```python
from build123d import *

# Parameters (mm, degrees)
SKETCH1_W             = 114.3
SKETCH1_H             = 25.4
SKETCH1_R             = 6.5
BOSS_EXTRUDE1_DEPTH   = 5.8
F_4_CLEARANCE_HOLE1_D = 2.9464
FILLET1_R             = 3.175


with BuildPart() as part:
    # Sketch1 → Boss-Extrude1 (new body)
    with BuildSketch(Plane(origin=(0, 0, 0), x_dir=(1, 0, 0), z_dir=(0, 1, 0))):
        with Locations((-57.15, 12.7)):
            Rectangle(SKETCH1_W, SKETCH1_H)
        with Locations(Location((-95.25, 12.7, 0), (0, 0, 270))):
            Circle(SKETCH1_R, mode=Mode.SUBTRACT)
        with Locations(Location((-57.15, 12.7, 0), (0, 0, 270))):
            Circle(SKETCH1_R, mode=Mode.SUBTRACT)
        with Locations(Location((-19.05, 12.7, 0), (0, 0, 270))):
            Circle(SKETCH1_R, mode=Mode.SUBTRACT)
    extrude(amount=BOSS_EXTRUDE1_DEPTH)

    # #4 Clearance Hole1 (through all)
    with Locations(Plane(origin=(0, 5.8, 0), x_dir=(-1, 0, 0), z_dir=(0, 1, 0))):
        with Locations((107.95, -22.225), (107.95, -3.175), (76.2, -22.225), (76.2, -3.175), (6.35, -22.225), (38.1, -22.225), (38.1, -3.175), (6.35, -3.175)):
            Hole(F_4_CLEARANCE_HOLE1_D / 2)

    # Fillet1
    fillet1_edges = [part.edges().sort_by_distance(p)[0] for p in [
        (0, 2.9, 0),
        (-114.3, 2.9, 0),
        (-114.3, 2.9, -25.4),
        (0, 2.9, -25.4),
    ]]
    fillet(fillet1_edges, radius=FILLET1_R)


solid = part.part
```
The listing builds one solid part. Answer for the finished solid, in the listing's coordinates (mm). Give positions to 0.01 mm unless a question says otherwise; leave off trailing zeros. Order: outer loops, then holes, each group sorted by start corner. A loop starts at its lowest first (then second) coordinate and runs counter-clockwise, first axis right, second up.
Item 1: The part is cut by section C-C, the plane z = -14. Give the vertices of the cut face in (x, y), and give its area (3 significant figures).
From the geometry:
outline: (-114.3, 0) - (-101.62, 0) - (-101.62, 5.8) - (-114.3, 5.8) - close; (-88.88, 0) - (-63.52, 0) - (-63.52, 5.8) - (-88.88, 5.8) - close; (-50.78, 0) - (-25.42, 0) - (-25.42, 5.8) - (-50.78, 5.8) - close; (-12.68, 0) - (0, 0) - (0, 5.8) - (-12.68, 5.8) - close
area: 441 mm2
Item 2: The part is cut by section D-D, the plane x = -97. Give the vertices of the cut face in (y, z).
From the geometry:
outline: (0, -25.4) - (5.8, -25.4) - (5.8, -18.96) - (0, -18.96) - close; (0, -6.44) - (5.8, -6.44) - (5.8, 0) - (0, 0) - close
Item 3: Find the intervals of material crossed by probe 1 along X at (y, z) = (1.65, -12.7); probe 2 along Z at (x, y) = (-6.35, 2.2); probe 3 along X at (y, z) = (5.3, -14.5), in increasing order.
From the geometry:
probe 1: x = -114.3 to -101.75, -88.75 to -63.65, -50.65 to -25.55, -12.55 to 0
probe 2: z = -25.4 to -23.7, -20.75 to -4.65, -1.7 to 0
probe 3: x = -114.3 to -101.5, -89 to -63.4, -50.9 to -25.3, -12.8 to 0
Item 4: For a pull along Z with two mould halves and no side action, classify faces 1 (the face through (0, 3, -13)), 2 (the face through (-7.82, 2.86, -3.11)), 3 (the face through (-58, 3, -25.4)) as pulls with the +Z half, pulls with the -Z half, needs draft (parallel to the pull), parting line crosses it, or undercut.
From the geometry:
face 1: needs draft
face 2: undercut
face 3: pulls with the -Z half
Item 5: The part is cut by section B-B, the plane y = 2. Count the separate pieces of the cut face and the enclosed holes in it, and give its area (3 significant figures).
From the geometry:
separate pieces: 1
enclosed holes: 11
area: 2,440 mm2
Item 6: The part is cut by section A-A, the plane x = -6.35. Give the vertices of the cut face in (y, z), and give its area (3 significant figures).
From the geometry:
outline: (0, -25.4) - (5.8, -25.4) - (5.8, -23.7) - (0, -23.7) - close; (0, -20.75) - (5.8, -20.75) - (5.8, -4.65) - (0, -4.65) - close; (0, -1.7) - (5.8, -1.7) - (5.8, 0) - (0, 0) - close
area: 113 mm2
